Geometry: see drawing. Coordinates: mm, zero at the bounding-box minimum. A direction names the side the tool comes from. Give positions to 0.01 mm unless a question says otherwise; leave off trailing zeros. Write each loop counter-clockwise with the first axis right and the second up, starting at its lowest first coordinate (ties: lowest second). Pieces come first, ordered by that corner, then holes. Notation, with made-up numbers: (-29, 84) - (25, 84) arc R7 ccw to (25, 90) - close; hole circle Ø8 at (51, 42.25). An arc over 180 degrees is marked (long way). Return JSON: item names as keys, results as strings.
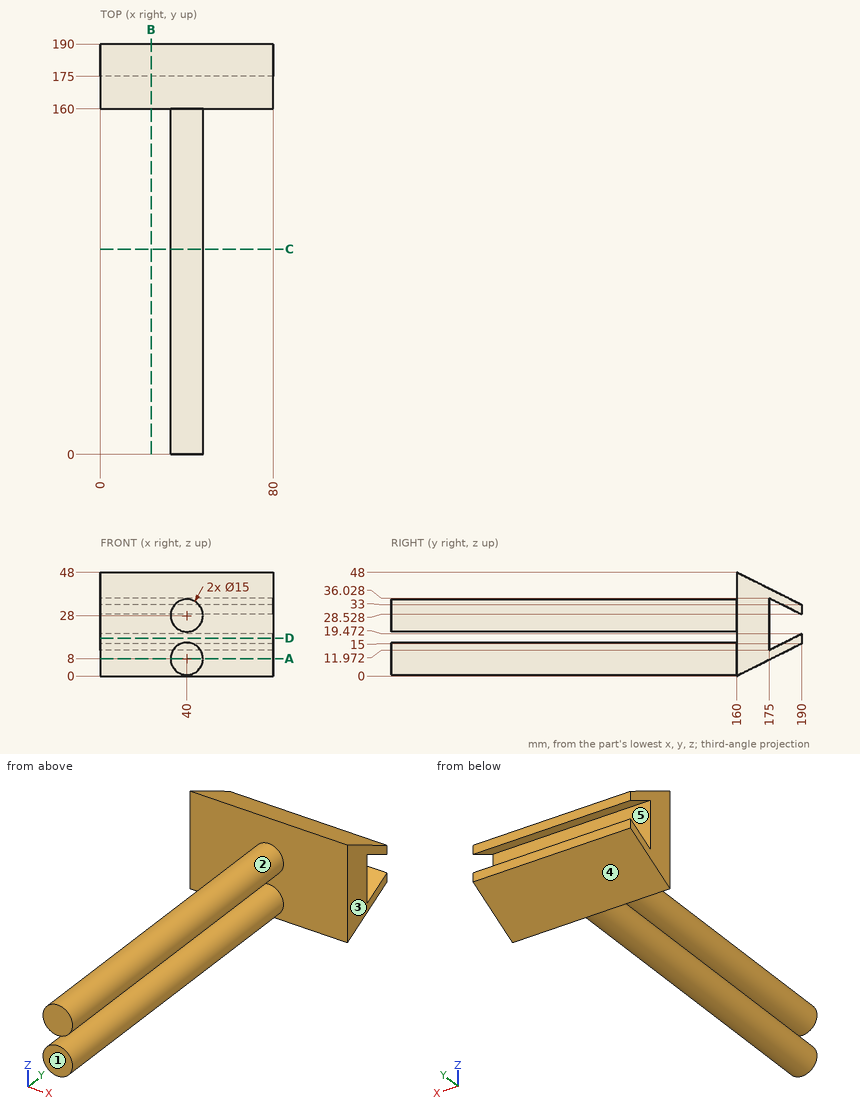
Q1. Section query A-A, the plane z = 8. Return the cut outline in (x, y).
Answer key:
{"outline": "(0, 160) - (32.5, 160) - (32.5, 0) - (47.5, 0) - (47.5, 160) - (80, 160) - (80, 176) - (0, 176) - close"}
Q2. Material intervals for probe 1 along Y at (x, z) = (23, 14.5) (1 decimal); probe 2 along Y at (x, z) = (65.5, 21.5); probe 3 along Y at (x, z) = (74.5, 18) (1 decimal), sorted ascending. Write a range as [from, to].
Answer key:
{"probe 1": "y = [160, 175], [180.1, 189]", "probe 2": "y = [160, 175]", "probe 3": "y = [160, 175], [187.1, 190]"}
Q3. Pin query (flat end, axial travel): P1, Ø4, axis at x = 42, y = 79, coming from the +Z side; P2, Ø12, axis at y = 129, z = 37.5, coming from the -X side; P3, Ø1, axis at x = 24.5, z = 27, coming from the +Y side. Return the tip coordinate at first contact, or that it passes through.
Answer key:
{"P1": "stops at z = 35.5", "P2": "stops at x = 33.37", "P3": "stops at y = 175"}
Q4. Section query B-B, the plane x = 23.5. Return the cut outline in (y, z), plus the area to 3 significant figures.
Answer key:
{"outline": "(160, 0) - (190, 15) - (190, 19.47) - (175, 11.97) - (175, 36.03) - (190, 28.53) - (190, 33) - (160, 48) - close", "area": "742 mm^2"}
Q5. Set-up query: the marked faces 1 and 2. Return all of +Z, -Z, +X, -X, +Y, -Y with unobstructed straight access to the full face (end or side cutting, diameter ignored); none if empty.
Answer key:
{"face 1": "+Z, -Z, +X, -X, -Y", "face 2": "-Y"}
Q6. Mould query, pull axis Z, two halves, no side actions, for the marked faces 3, 4 and 5. Classes: pulls with the +Z half, pulls with the -Z half, needs draft (parallel to the pull), parting line crosses it, or undercut.
Answer key:
{"face 3": "needs draft", "face 4": "pulls with the -Z half", "face 5": "undercut"}
Q7. Section query D-D, the plane z = 17.5. Return the cut outline in (x, y).
Answer key:
{"outline": "(0, 160) - (80, 160) - (80, 175) - (0, 175) - close; (0, 186.06) - (80, 186.06) - (80, 190) - (0, 190) - close"}
Q8. Section query C-C, the plane y = 95. Return the cut outline in (x, z), plus the area to 3 significant figures.
Answer key:
{"outline": "circle Ø15 at (40, 8); circle Ø15 at (40, 28)", "area": "353 mm^2"}
